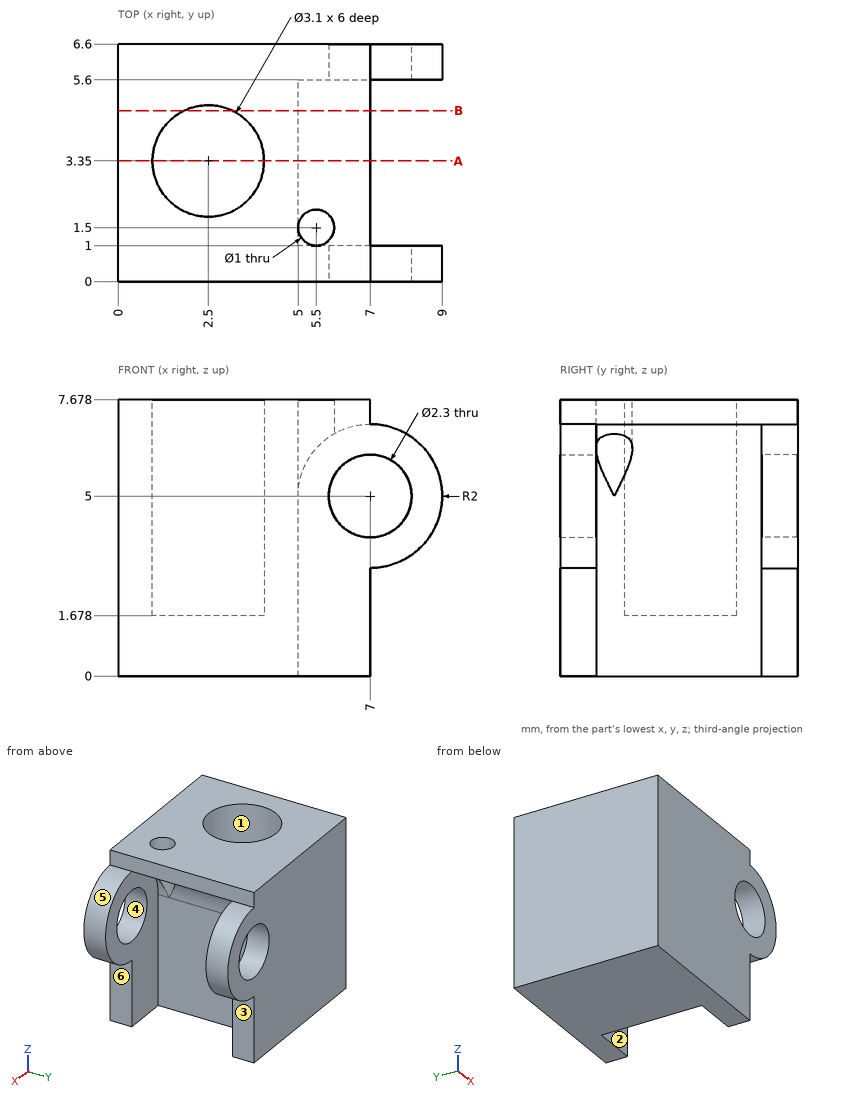
Input: dimensioned drawing with shaded views. Units: mm. Origin: part minimum x, y, z. A direction names the side the tool comes from. Round coordinates to 2 decimals unless told otherwise and drop trailing zeros. Loops run counter-clockwise (first coordinate to the right, second up) from the corner with the lowest first, then second, coordinate; pieces in that order, holes last. Notation, with made-up numbers: (8.25, 86.25) -> (14.25, 86.25) arc R26 cw to (14.25, 103.25) -> close; hole circle Ø5 at (8.5, 69). An arc over 180 degrees is marked (long way). Answer as a JSON object with one key per item and string values. Group by question number.
1) Pin query (flat end, axial travel): pin 1 (1.4 mm diameter, centred on y = 3, z = 3.5, fed in from +X); pin 2 (3 mm diameter, centred on y = 1.5, z = 3, fed in from +X); pin 3 (1.1 mm diameter, centred on y = 6, z = 1, fed in from +X). Return the tip coordinate at first contact, or that it passes through.
2) Section query B-B on y = 4.75. Output: boundary loops of the cut face in (x, z) (1 decimal).
3) Draft query along Z for the marked faces 4, 5 and 6. Return one class per face: +Z half, -Z half, draft (parallel to the pull), parting line (faces both ways), or undercut.
4) Ray query, L1, parallel to Y at x = 5.5, z = 3.5; L2, parallel to Y at x = 2.5, z = 4.8; L3, parallel to X at y = 3.35, z = 4.4. Return the intervals inside material, ascending.
5) Reachability of the marked faces 1, 2 and 3 from +Z, -Z, +X, -X, +Y, -Y: full face, straight path, thin tool, end or side. Return the list, or none.
6) Section query A-A on y = 3.35. Output: boundary loops of the cut face in (x, z), plus the area to 3 significant figures.
Reply:
{
 "1": {"pin 1": "stops at x = 5", "pin 2": "stops at x = 8.91", "pin 3": "stops at x = 7"},
 "2": {"outline": "(0, 0) -> (5, 0) -> (5, 5) arc R2 cw to (7, 7) -> (7, 7.7) -> (3.2, 7.7) -> (3.2, 1.7) -> (1.8, 1.7) -> (1.8, 7.7) -> (0, 7.7) -> close"},
 "3": {"face 4": "undercut", "face 5": "parting line", "face 6": "draft"},
 "4": {"L1": "y = 0 to 1, 5.6 to 6.6", "L2": "y = 0 to 1.8, 4.9 to 6.6", "L3": "x = 0 to 0.95, 4.05 to 5"},
 "5": {"face 1": "+Z", "face 2": "-Z, +X", "face 3": "-Z, +X, +Y, -Y"},
 "6": {"outline": "(0, 0) -> (5, 0) -> (5, 5) arc R2 cw to (7, 7) -> (7, 7.68) -> (4.05, 7.68) -> (4.05, 1.68) -> (0.95, 1.68) -> (0.95, 7.68) -> (0, 7.68) -> close", "area": "22.0 mm2"}
}
